Geometry check sheet. Reference: the model listing, model coordinates, mm. A direction names the side the tool comes from. Give positions to 0.01 mm unless a question says otherwise; leave off trailing zeros. Order: outer loops, then holes, each group sorted by start corner. A loop starts at its lowest first (then second) coordinate and runs counter-clockwise, first axis right, second up. Notation, with made-up numbers: (69, 80.5) - (119, 80.5) arc R30 ccw to (119, 116.5) - close; hole circle Ø6 at (46, 46.5). An arc over 180 degrees is marked (long way). Put each result on its own line as item: value. Start each with the question number.
Autodesk Inventor part; units mm, degrees
ref_plane "YZ Plane" through (0, 0, 0) normal (1, 0, 0) x (0, 1, 0)
ref_plane "XZ Plane" through (0, 0, 0) normal (0, 1, 0) x (-1, 0, 0)
ref_plane "XY Plane" through (0, 0, 0) normal (0, 0, 1) x (1, 0, 0)
sketch "スケッチ1" plane through (0, 0, 0) normal (0, 0, 1) x (1, 0, 0)
  line L0 (0, 0) -> (30, 0)
  line L1 (30, 0) -> (30, 5)
  line L2 (30, 5) -> (15, 20)
  line L3 (15, 20) -> (0, 20)
  line L4 (0, 20) -> (0, 0)
  dimension "d0" = 20
  dimension "d1" = 30
  dimension "d2" = 15
  dimension "d3" = 5
extrude "押し出し1" add sketch "スケッチ1" along normal blind 20
sketch "スケッチ2" plane through (0, 20, 0) normal (0, 1, 0) x (1, 0, 0)
  line L0 (4.4, -3) -> (30, -3)
  line L1 (30, -3) -> (30, -17)
  line L2 (30, -17) -> (4.4, -17)
  line L3 (4.4, -17) -> (4.4, -3)
  line L4 (15, 0) -> (0, 0)
  line L5 (15, -20) -> (0, -20)
  line L6 (0, 0) -> (0, -20)
  line L7 (30, 0) -> (30, -20)
  dimension "d7" = 3
  dimension "d8" = 3
  dimension "d9" = 4.4
extrude "押し出し2" cut sketch "スケッチ2" against normal blind 15.6
chamfer "面取り1" distance 2 angle 45 2 edges at (4.4, 20, 10) (30, 4.4, 10)
sketch "スケッチ3" plane through (0, 0, 0) normal (-1, 0, 0) x (0, 0, 1)
  line L0 (0, 0) -> (20, 0) construction
  line L1 (10, 0) -> (10, 20) construction
  line L2 (0, 20) -> (20, 20) construction
  line L3 (0, 5) -> (0, 20) construction
  circle A0 centre (10, 10) radius 2.5
  dimension "d15" = 5
extrude "押し出し3" cut sketch "スケッチ3" against normal through all
sketch "スケッチ4" plane through (0, 0, 0) normal (0, -1, 0) x (1, 0, 0)
  line L0 (30, 0) -> (30, 20) construction
  line L1 (30, 10) -> (0, 10) construction
  circle A0 centre (18, 10) radius 2.5
  point P0 (0, 0)
  dimension "d18" = 5
  dimension "d19" = 12
extrude "押し出し4" cut sketch "スケッチ4" against normal up to next
properties part number "ブラケット"
Item 1: Set-up check for faces 1 (the face through (0, 12, 8)), 2 (the face through (13, 11, 17)): record each of +Z, -Z, +X, -X, +Y, -Y from which the full face is reachable in a straight line by a thin tool's end or side.
Item 2: Thickness scan on line 1 along Y through (x, z) = (2.1, 10); line 2 along Z through (x, y) = (13, 15.5). Record the ranges inside material, lowest first.
Item 3: Cross-section at C-C (y = 10). Enter the section's corners in (x, z), and give its area (3 significant figures).
Item 4: Cross-section at A-A (x = 16). Enter the section's corners in (y, z).
Item 5: Cross-section at D-D (x = 27). Enter the section's corners in (y, z), and give its area (3 significant figures).
Item 6: Release check for a two-part mould opening along Z. For faces 3 (the face through (11, 10, 20)), 4 (the face through (16, 4.4, 8)), 5 (the face through (3.4, 19, 10.1)), 6 (the face through (30, 1, 10)) record: +Z half, -Z half, draft (parallel to the pull), parting line (faces both ways), or undercut.
Item 7: Cross-section at B-B (z = 10). Enter the section's corners in (x, y), and give its area (3 significant figures).
Item 8: Gauge pin test, flat ends, axial feed: pin 1 Ø3 at (x, z) = (13.5, 8) entering from +Y; pin 2 Ø4 at (y, z) = (10, 10) entering from -X; pin 3 Ø6 at (y, z) = (14.5, 16.5) entering from +X. Record the tip position at first contact, or that the pin passes through.
Recorded:
1. face 1: +Z, -Z, -X, +Y, -Y
1. face 2: +X, +Y
2. line 1: y = 0 to 7.5, 12.5 to 20
2. line 2: z = 0 to 3, 17 to 20
3. outline: (0, 0) - (25, 0) - (25, 3) - (4.4, 3) - (4.4, 7.5) - (0, 7.5) - close; (0, 12.5) - (4.4, 12.5) - (4.4, 17) - (25, 17) - (25, 20) - (0, 20) - close
3. area: 190 mm^2
4. outline: (0, 0) - (19, 0) - (19, 3) - (4.4, 3) - (4.4, 8.5) - (0, 8.5) - close; (0, 11.5) - (4.4, 11.5) - (4.4, 17) - (19, 17) - (19, 20) - (0, 20) - close
5. outline: (0, 0) - (8, 0) - (8, 3) - (4.4, 3) - (4.4, 17) - (8, 17) - (8, 20) - (0, 20) - close
5. area: 110 mm^2
6. face 3: +Z half
6. face 4: undercut
6. face 5: undercut
6. face 6: draft
7. outline: (0, 0) - (15.5, 0) - (15.5, 4.4) - (4.4, 4.4) - (4.4, 7.5) - (0, 7.5) - close; (0, 12.5) - (4.4, 12.5) - (4.4, 18) - (2.4, 20) - (0, 20) - close; (20.5, 0) - (30, 0) - (30, 2.4) - (28, 4.4) - (20.5, 4.4) - close
7. area: 153 mm^2
8. pin 1: stops at y = 4.4
8. pin 2: passes through
8. pin 3: stops at x = 23.46
